Check sheet for the modelled part. Datum: model origin and axes. Units: mm. Round coordinates to 2 decimals unless told otherwise and drop trailing zeros. Loops run counter-clockwise (first coordinate to the right, second up) from the corner with the lowest first, then second, coordinate; pieces in that order, holes last. Notation, with made-up numbers: (-35, 12.25) - (-6, 12.25) arc R20 cw to (-6, 41.25) - close; hole circle Ø5 at (-19.5, -28.5). An arc over 180 degrees is marked (long way). Answer in a Markdown table with one row per item. Add a question column.
(1) Cross-section at A-A on z = 1374.5. Enter the section's corners in (x, y).
(2) Thickness scan on line 1 along X through (y, z) = (22, 1087.5); line 2 along Z through (x, y) = (-96, 41); line 3 along Y through (x, z) = (-185.5, 1104.5). Record the ranges inside material, lowest first.
(3) Gauge pin test, flat ends, axial feed: pin 1 (12 mm diameter, centred on x = -212.5, z = 654, fed in from -Y); pin 2 (12 mm diameter, centred on y = 63.5, z = 1427.5, fed in from +X); pin 3 (12 mm diameter, centred on x = -174, y = 37, fed in from +Z). Record the tip position at first contact, or that the pin passes through.
from build123d import *

# Parameters (mm, degrees)
F1_DEPTH = 1803.4
F2_T     = -30


with BuildPart() as f1:
    # F0 (on Top) → F1 (new body)
    with BuildSketch(Plane.XY):
        Polygon((-58.050863, -69.46938), (-29.354431, -21.759306), (-28.35763, 33.907045), (-55.32755, 82.613921), (-103.037623, 111.310352), (-158.703975, 112.307154), (-207.41085, 85.337233), (-236.107282, 37.62716), (-237.104083, -18.039192), (-210.134163, -66.746067), (-162.42409, -95.442498), (-106.757738, -96.4393), align=None)
    extrude(amount=F1_DEPTH)

    # F2
    f2_openings = [f1.faces().sort_by_distance(p)[0] for p in [
        (-43.702647, -45.614343, 901.7),
        (-132.730857, 7.933927, 1803.4),
    ]]
    offset(amount=F2_T, openings=f2_openings)


solid = f1.part
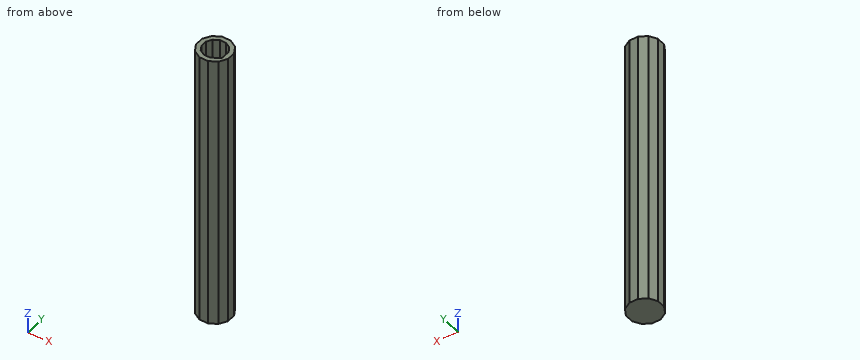
Answers:
| question | item | result |
|---|---|---|
| 1 | outline | (-237.1, -18.04) - (-210.13, -66.75) - (-162.42, -95.44) - (-106.76, -96.44) - (-58.05, -69.47) - (-29.35, -21.76) - (-28.36, 33.91) - (-55.33, 82.61) - (-103.04, 111.31) - (-158.7, 112.31) - (-207.41, 85.34) - (-236.11, 37.63) - close; hole (-206.96, -10.54) - (-187.78, -45.18) - (-153.85, -65.59) - (-114.26, -66.3) - (-59.62, -36.04) - (-58.5, 26.41) - (-77.68, 61.05) - (-111.61, 81.46) - (-151.2, 82.17) - (-185.85, 62.99) - (-206.26, 29.05) - close |
| 2 | line 1 | x = -236.39 to -206.38, -58.58 to -28.57 |
| 2 | line 2 | z = 0 to 30 |
| 2 | line 3 | y = -81.56 to -46.55, 63.18 to 97.47 |
| 3 | pin 1 | stops at y = -68.93 |
| 3 | pin 2 | stops at x = -41.42 |
| 3 | pin 3 | stops at z = 30 |
